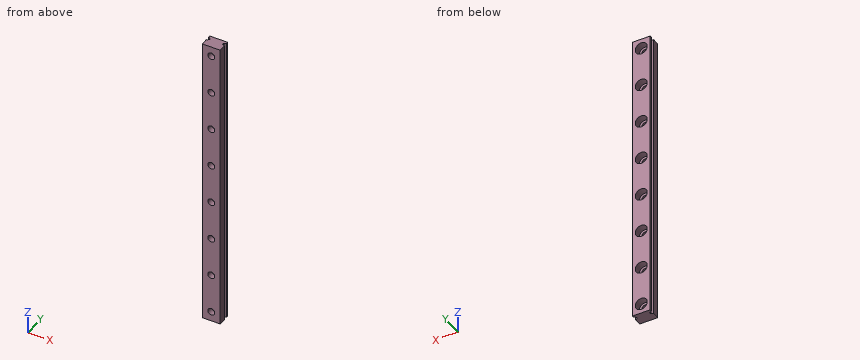
```python
from build123d import *

# Parameters (mm, degrees)
EXTRUDE1_DEPTH  = 150
SKETCH2_R       = 3
EXTRUDE2_DEPTH  = 3.5
SKETCH_R        = 1.75
EXTRUDE3_DEPTH  = 7.5
LPATTERN1_COUNT = 13
LPATTERN1_PITCH = 20


with BuildPart() as part:
    # Sketch1 → Extrude1 (new body)
    with BuildSketch(Plane.XY):
        with BuildLine():
            Line((-4.5, -3.25), (4.5, -3.25))
            Line((4.5, -3.25), (4.5, 0.25))
            ThreePointArc((4.5, 0.25), (3.93077967, 0.427814974), (3.563991137, 0.898023568))
            Line((3.563991137, 0.898023568), (3.235073025, 0.898023568))
            Line((3.235073025, 0.898023568), (3.235073025, 1.601976432))
            Line((3.235073025, 1.601976432), (3.563991137, 1.601976432))
            ThreePointArc((3.563991137, 1.601976432), (3.93077967, 2.072185026), (4.5, 2.25))
            Line((4.5, 2.25), (4.5, 3.25))
            Line((4.5, 3.25), (-4.5, 3.25))
            Line((-4.5, 3.25), (-4.5, 2.25))
            ThreePointArc((-4.5, 2.25), (-3.93077967, 2.072185026), (-3.563991137, 1.601976432))
            Line((-3.563991137, 1.601976432), (-3.235073025, 1.601976432))
            Line((-3.235073025, 1.601976432), (-3.235073025, 0.898023568))
            Line((-3.235073025, 0.898023568), (-3.563991137, 0.898023568))
            ThreePointArc((-3.563991137, 0.898023568), (-3.93077967, 0.427814974), (-4.5, 0.25))
            Line((-4.5, 0.25), (-4.5, -3.25))
        make_face()
    extrude(amount=EXTRUDE1_DEPTH)

    # Sketch2 → Extrude2 (cut)
    with BuildSketch(Plane(origin=(0, 3.25, 0), x_dir=(1, 0, 0), z_dir=(0, 1, 0))):
        with Locations((0, -5)):
            Circle(SKETCH2_R)
    extrude2 = extrude(amount=-EXTRUDE2_DEPTH, mode=Mode.SUBTRACT)

    # Sketch → Extrude3 (cut, through all)
    with BuildSketch(Plane(origin=(0, 3.25, 0), x_dir=(1, 0, 0), z_dir=(0, 1, 0))):
        with Locations((0, -5)):
            Circle(SKETCH_R)
    extrude3 = extrude(amount=-EXTRUDE3_DEPTH, mode=Mode.SUBTRACT)

    # LPattern1: Extrude2, Extrude3 ×13
    with Locations(*[(0, 0, i * LPATTERN1_PITCH) for i in range(1, LPATTERN1_COUNT)]):
        add(extrude2, mode=Mode.SUBTRACT)
        add(extrude3, mode=Mode.SUBTRACT)


solid = part.part
```
Geometry check sheet. Reference: the model listing, model coordinates, mm. Coordinates: 2 decimals unless noted, no trailing zeros. Order: outer loops, then holes, each group sorted by start corner. A loop starts at its lowest first (then second) coordinate and runs counter-clockwise, first axis right, second up.
Q1. Depth check by flat-ended pin: pin 1 Ø5 at (x, z) = (0, 25) entering from +Y; pin 2 Ø3 at (x, z) = (0, 5) entering from -Y. Enter the tip coordinate at first touch or a pass-through.
Reply:
pin 1: stops at y = -0.25
pin 2: passes through
Q2. Sectioned sample at A-A on z = 65. Record the cut outline in (x, y), and give its area (3 significant figures).
Reply:
outline: (-4.5, -3.25) - (-1.75, -3.25) - (-1.75, -0.25) - (-3, -0.25) - (-3, 3.25) - (-4.5, 3.25) - (-4.5, 2.25) arc R1 cw to (-3.56, 1.6) - (-3.24, 1.6) - (-3.24, 0.9) - (-3.56, 0.9) arc R1 cw to (-4.5, 0.25) - close; (1.75, -3.25) - (4.5, -3.25) - (4.5, 0.25) arc R1 cw to (3.56, 0.9) - (3.24, 0.9) - (3.24, 1.6) - (3.56, 1.6) arc R1 cw to (4.5, 2.25) - (4.5, 3.25) - (3, 3.25) - (3, -0.25) - (1.75, -0.25) - close
area: 23.5 mm2
Q3. Sectioned sample at B-B on y = -1.75. Give the number of separate pieces and of enclosed holes in the cut face, and give its area (3 significant figures).
Reply:
separate pieces: 1
enclosed holes: 8
area: 1,270 mm2
Q4. Sectioned sample at C-C on z = 110.5. Record the cut outline in (x, y), and give its area (3 significant figures).
Reply:
outline: (-4.5, -3.25) - (4.5, -3.25) - (4.5, 0.25) arc R1 cw to (3.56, 0.9) - (3.24, 0.9) - (3.24, 1.6) - (3.56, 1.6) arc R1 cw to (4.5, 2.25) - (4.5, 3.25) - (-4.5, 3.25) - (-4.5, 2.25) arc R1 cw to (-3.56, 1.6) - (-3.24, 1.6) - (-3.24, 0.9) - (-3.56, 0.9) arc R1 cw to (-4.5, 0.25) - close
area: 55.0 mm2
Q5. Thickness scan on probe 1 along X at (y, z) = (1.3, 65); probe 2 along X at (y, z) = (-2, 45); probe 3 along Y at (x, z) = (2.25, 103.5). Record the ranges inside material, lowest first.
Reply:
probe 1: x = -3.24 to -3, 3 to 3.24
probe 2: x = -4.5 to -1.75, 1.75 to 4.5
probe 3: y = -3.25 to -0.25
